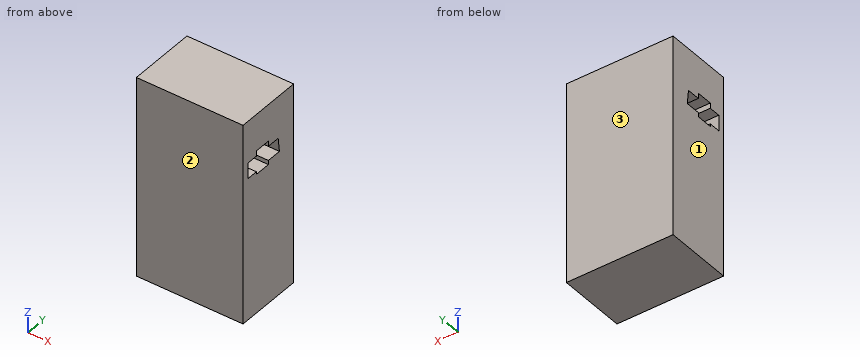
Autodesk Inventor part; units mm, degrees
ref_plane "YZ Plane" through (0, 0, 0) normal (1, 0, 0) x (0, 1, 0)
ref_plane "XZ Plane" through (0, 0, 0) normal (0, 1, 0) x (-1, 0, 0)
ref_plane "XY Plane" through (0, 0, 0) normal (0, 0, 1) x (1, 0, 0)
sketch "Sketch1" plane through (0, 0, 0) normal (1, 0, 0) x (0, 1, 0)
  line L0 (10.9667, -32.2396) -> (-10.9667, -32.2396)
  line L1 (-10.9667, -32.2396) -> (-10.9667, 32.2396)
  line L2 (-10.9667, 32.2396) -> (10.9667, 32.2396)
  line L3 (10.9667, 32.2396) -> (10.9667, -32.2396)
  line L4 (10.9667, -32.2396) -> (-10.9667, 32.2396) construction
  line L5 (-10.9667, -32.2396) -> (10.9667, 32.2396) construction
  line L6 (-8.867, 14.9521) -> (-8.867, 18.6958)
  line L7 (-8.867, 18.6958) -> (-5.1781, 18.6958)
  line L8 (-5.1781, 18.6958) -> (-5.1781, 20.3884)
  line L9 (-5.1781, 20.3884) -> (0.0187, 20.3884)
  line L10 (0.0187, 20.3884) -> (0.0187, 18.6958)
  line L11 (0.0187, 18.6958) -> (4.2724, 18.6958)
  line L12 (4.2724, 18.6958) -> (4.8008, 14.1133)
  line L13 (4.8008, 14.1133) -> (0.0187, 14.1133)
  line L14 (0.0187, 14.1133) -> (0.0187, 12.7771)
  line L15 (0.0187, 12.7771) -> (-5.1781, 12.7771)
  line L16 (-5.1781, 12.7771) -> (-5.1781, 13.6309)
  line L17 (-5.1781, 13.6309) -> (-8.867, 13.6309)
  line L18 (-8.867, 13.6309) -> (-8.867, 14.9521)
  point P0 (0, 0)
extrude "Extrusion1" add sketch "Sketch1" along normal blind 34.25
properties part number "test blok"
The model under review builds one solid part; all positions refer to its coordinate system, in mm. Face numbers are marked on the shaded views. Round coordinates to 2 decimals unless told otherwise and drop trailing zeros. Write each loop counter-clockwise with the first axis right and the second up, starting at its lowest first coordinate (ties: lowest second). Pieces come first, ordered by that corner, then holes. Notation, with made-up numbers: (-30.5, 30.5) -> (6.5, 30.5) arc R25 ccw to (6.5, 61.5) -> close; hole circle Ø2 at (-35.75, 38.25). An arc over 180 degrees is marked (long way). Use CSV: the item, a comma, the result in double quotes.
Q1. To check wall thickness, follow probe 1 along Z at (x, y) = (18, -8); probe 2 along Z at (x, y) = (4.5, 0.75); probe 3 along Y at (x, z) = (5, 14.5). State the ranges of each line that lie inside material, in increasing order. Write a range as [from, to].
Checks:
probe 1,"[-32.24, 13.63], [18.7, 32.24]"
probe 2,"[-32.24, 14.11], [18.7, 32.24]"
probe 3,"[-10.97, -8.87], [4.76, 10.97]"
Q2. Consider section B-B (x = 13). Give the boundary of the cut face in (y, z), then the cut area to 3 significant figures.
Checks:
outline,"(-10.97, -32.24) -> (10.97, -32.24) -> (10.97, 32.24) -> (-10.97, 32.24) -> close; hole (-8.87, 13.63) -> (-5.18, 13.63) -> (-5.18, 12.78) -> (0.02, 12.78) -> (0.02, 14.11) -> (4.8, 14.11) -> (4.27, 18.7) -> (0.02, 18.7) -> (0.02, 20.39) -> (-5.18, 20.39) -> (-5.18, 18.7) -> (-8.87, 18.7) -> close"
area,"1,340 mm²"
Q3. Consider section C-C (y = 3.25). Give the boundary of the cut face in (x, z).
Checks:
outline,"(0, -32.24) -> (34.25, -32.24) -> (34.25, 14.11) -> (0, 14.11) -> close; (0, 18.7) -> (34.25, 18.7) -> (34.25, 32.24) -> (0, 32.24) -> close"
Q4. Mouldability with a two-part tool opening along Y and no side actions: class the marked faces 1, 2 and 3 as released by +Y, released by -Y, zero draft, split by the parting line, or undercut.
Checks:
face 1,"zero draft"
face 2,"released by -Y"
face 3,"released by +Y"
Q5. Consider section A-A (y = -1). Give the boundary of the cut face in (x, z).
Checks:
outline,"(0, -32.24) -> (34.25, -32.24) -> (34.25, 12.78) -> (0, 12.78) -> close; (0, 20.39) -> (34.25, 20.39) -> (34.25, 32.24) -> (0, 32.24) -> close"
